from build123d import *

# Parameters (mm, degrees)
BOSS_EXTRUDE1_DEPTH = 6.35
SKETCH2_R           = 6.35
SKETCH2_R_2         = 5.08
BOSS_EXTRUDE2_DEPTH = 12.7
BOSS_EXTRUDE3_START = 5.08
BOSS_EXTRUDE3_DEPTH = 2.54
FILLET1_R           = 1.27


with BuildPart() as part:
    # Sketch1 → Boss-Extrude1 (new body)
    with BuildSketch(Plane(origin=(0, 0, 0), x_dir=(1, 0, 0), z_dir=(0, 1, 0))):
        with BuildLine():
            Line((0, 0), (-38.1, 0))
            ThreePointArc((-38.1, 0), (-65.040768363, -65.040768363), (0, -38.1))
            Line((0, -38.1), (0, 0))
        make_face()
    extrude(amount=BOSS_EXTRUDE1_DEPTH)

    # Sketch2 → Boss-Extrude2 (add)
    with BuildSketch(Plane(origin=(0, 6.35, 0), x_dir=(1, 0, 0), z_dir=(0, 1, 0))):
        with Locations(Location((-7.62, -7.62, 0), (0, 0, 270))):
            Circle(SKETCH2_R)
        with Locations(Location((-7.62, -7.62, 0), (0, 0, 270))):
            Circle(SKETCH2_R_2, mode=Mode.SUBTRACT)
    extrude(amount=BOSS_EXTRUDE2_DEPTH)

    # Sketch3 → Boss-Extrude3 (add)
    with BuildSketch(Plane(origin=(0, 6.35, 0), x_dir=(1, 0, 0), z_dir=(0, 1, 0)).offset(BOSS_EXTRUDE3_START)):
        with BuildLine():
            Line((-9.216562761, -2.797408648), (-8.563437239, -3.928655235))
            ThreePointArc((-8.563437239, -3.928655235), (-7.62, -3.81), (-6.676562761, -3.928655235))
            Line((-6.676562761, -3.928655235), (-6.023437239, -2.797408648))
            ThreePointArc((-6.023437239, -2.797408648), (-7.62, -2.54), (-9.216562761, -2.797408648))
        make_face()
        with BuildLine():
            ThreePointArc((-6.676562761, -11.311344765), (-7.62, -11.43), (-8.563437239, -11.311344765))
            Line((-8.563437239, -11.311344765), (-9.216562761, -12.442591352))
            ThreePointArc((-9.216562761, -12.442591352), (-7.62, -12.7), (-6.023437239, -12.442591352))
            Line((-6.023437239, -12.442591352), (-6.676562761, -11.311344765))
        make_face()
    extrude(amount=BOSS_EXTRUDE3_DEPTH)

    # Fillet1
    fillet1_edges = [part.edges().sort_by_distance(p)[0] for p in [
        (-65.040768363, 6.35, 65.040768363),
        (0, 6.35, 19.05),
        (-19.05, 6.35, 0),
    ]]
    fillet(fillet1_edges, radius=FILLET1_R - 0.0001)  # a hair under: the kernel refuses the full size


solid = part.part
Could you check a few things on this model? Use its own coordinates, in mm. A direction names the side the tool comes from. Give positions to 0.01 mm unless a question says otherwise; leave off trailing zeros. Order: outer loops, then holes, each group sorted by start corner. A loop starts at its lowest first (then second) coordinate and runs counter-clockwise, first axis right, second up. Notation, with made-up numbers: (25.5, 46) - (60.5, 46) arc R14 cw to (60.5, 65) - close; hole circle Ø7 at (78.5, 67.25). An arc over 180 degrees is marked (long way). Return JSON: item names as keys, results as strings. Group by question number.
Q1. Which directions (+Z, -Z, +X, -X, +Y, -Y) give clear straight access to the entire face, cutting with the end or side of a thin tool? Please do faces 1 (the face through (0, 3, 19)), 2 (the face through (-7.61, 12.68, 11.43)).
Q2. Thinking about a two-plate mould opening in X: for faces 3 (the face through (-7.63, 12.68, 3.81)), 4 (the face through (-8, 6.35, 8)), 5 (the face through (-11.48, 12.61, 2.58)), 6 (the face through (-3, 19.05, 5)), which applies, pulls with the +X half, pulls with the -X half, needs draft (parallel to the pull), parting line crosses it, or undercut?
Q3. Please list where these lines run through material, in increasing order: line 1 along X through (y, z) = (11, 7.62); line 2 along Y through (x, z) = (-27.5, 5.5); line 3 along Z through (x, y) = (-10, 14.25). Write a range as [from, to].
Q4. Will these pins go through, and if not, where does the flat tip stop? pin 1 Ø1.5 at (y, z) = (5, 56) entering from +X; pin 2 Ø6 at (x, z) = (-39, 56.5) entering from +Y; pin 3 Ø8 at (y, z) = (12, 17) entering from +X.
Q5. Suppose I cut it at A-A, the plane y = 12.75. Please give me the cut outline in (x, z).
Resolved:
{
 "1": {"face 1": "+Z, -Z, +X, +Y, -Y", "face 2": "+Y"},
 "2": {"face 3": "undercut", "face 4": "undercut", "face 5": "parting line crosses it", "face 6": "needs draft"},
 "3": {"line 1": "x = [-13.97, -12.7], [-2.54, -1.27]", "line 2": "y = [0, 6.35]", "line 3": "z = [1.73, 3.13], [12.11, 13.51]"},
 "4": {"pin 1": "stops at x = -4.08", "pin 2": "stops at y = 6.35", "pin 3": "stops at x = -4.25"},
 "5": {"outline": "circle Ø12.7 at (-7.62, 7.62); hole (-9.22, 2.8) - (-8.56, 3.93) arc R3.81 ccw to (-6.68, 3.93) - (-6.02, 2.8) arc R5.08 ccw to (-6.02, 12.44) - (-6.68, 11.31) arc R3.81 ccw to (-8.56, 11.31) - (-9.22, 12.44) arc R5.08 ccw to start"}
}
